Answer from the drawing. Dimensions are ordinates in mm from the lowest x, y and z of the part. A direction names the side the tool comes from. Coordinates: 2 decimals unless noted, no trailing zeros. Write each loop counter-clockwise with the first axis right and the second up, starting at its lowest first coordinate (ties: lowest second). Pieces come first, ordered by that corner, then holes.
(1) Given pin 1 (11.5 mm diameter, centred on x = 20.5, z = 30.5, fed in from +Y); pin 2 (1 mm diameter, centred on y = 6, z = 31, fed in from -X); pin 3 (3 mm diameter, centred on x = 19, y = 6.5, fed in from +Z); pin 4 (12 mm diameter, centred on x = 33.5, z = 31, fed in from -Y), each flat-ended and moving along its own axis, determine where each tip first touches the part or whether it passes through.
(2) Section A-A on x = 6.9 is taken. Write down the section's boundary in (y, z).
(3) Section B-B on z = 31 is taken. Write down the section's boundary in (x, y), then the cut area to 3 significant figures.
(4) Section C-C on x = 21.5 is taken. Write down the section's boundary in (y, z), then the cut area to 3 significant figures.
(5) The mould has two halves that part along X. Classify the marked faces 4, 5, 6 and 7: +X half, -X half, draft (parallel to the pull), parting line (faces both ways), or undercut.
(6) Which of the six approach directions +Z, -Z, +X, -X, +Y, -Y give full straight-line access (tool end or side, diameter ignored) to the marked faces 1, 2 and 3?
(7) Find the intervals of material crossed by probe 1 along Y at (x, z) = (45.4, 24.3); probe 2 along Y at (x, z) = (6, 24); probe 3 along Y at (x, z) = (15, 38.5), in increasing order.
(8) Section D-D on y = 23 is taken. Write down the section's boundary in (x, z).
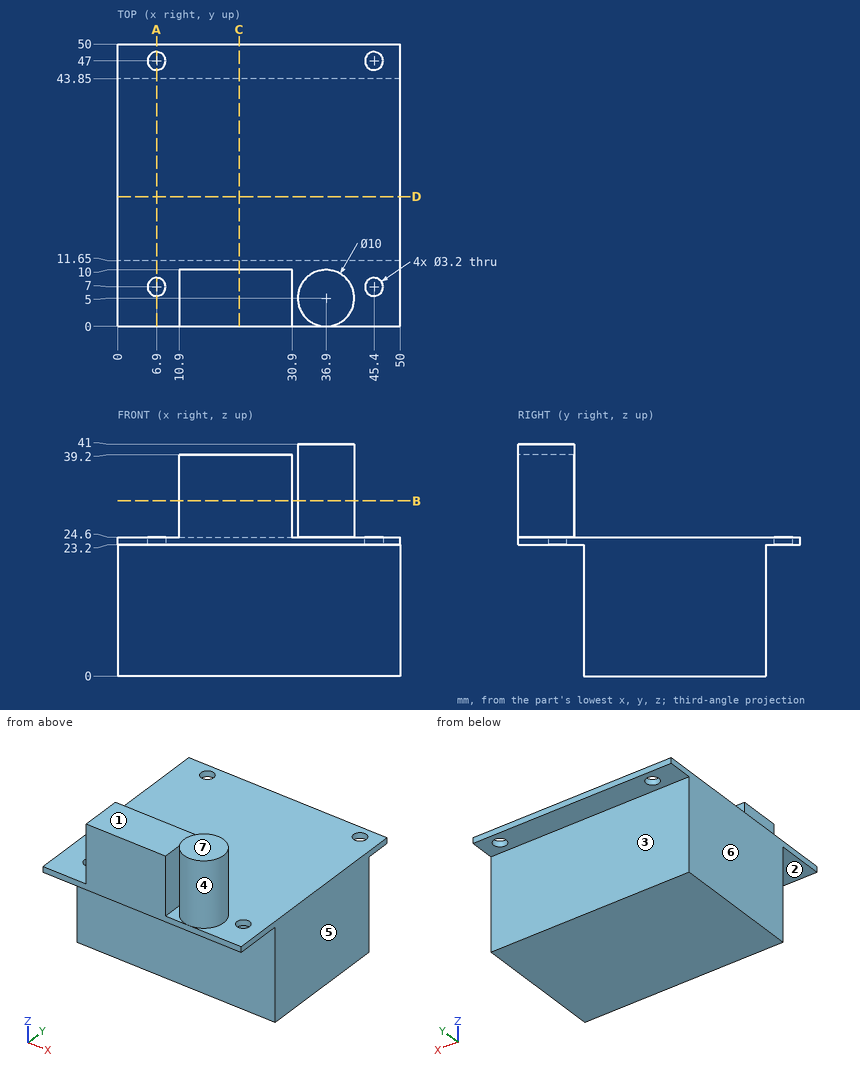
Response:
1. pin 1: stops at y = 10
1. pin 2: stops at x = 10.9
1. pin 3: stops at z = 39.2
1. pin 4: stops at y = 0
2. outline: (0, 23.2) - (5.4, 23.2) - (5.4, 24.6) - (0, 24.6) - close; (8.6, 23.2) - (11.65, 23.2) - (11.65, 0) - (43.85, 0) - (43.85, 23.2) - (45.4, 23.2) - (45.4, 24.6) - (8.6, 24.6) - close; (48.6, 23.2) - (50, 23.2) - (50, 24.6) - (48.6, 24.6) - close
3. outline: (10.9, 0) - (30.9, 0) - (30.9, 10) - (10.9, 10) - close; circle Ø10 at (36.9, 5)
3. area: 279 mm2
4. outline: (0, 23.2) - (11.65, 23.2) - (11.65, 0) - (43.85, 0) - (43.85, 23.2) - (50, 23.2) - (50, 24.6) - (10, 24.6) - (10, 39.2) - (0, 39.2) - close
4. area: 963 mm2
5. face 4: undercut
5. face 5: +X half
5. face 6: -X half
5. face 7: draft
6. face 1: +Z, -X, +Y, -Y
6. face 2: -Z, +X, -X, -Y
6. face 3: -Z, +X, -X, +Y
7. probe 1: y = 0 to 5.4, 8.6 to 45.4, 48.6 to 50
7. probe 2: y = 0 to 5.68, 8.32 to 45.68, 48.32 to 50
7. probe 3: y = 0 to 10
8. outline: (0, 0) - (50, 0) - (50, 24.6) - (0, 24.6) - close
